```python
from build123d import *

# Parameters (mm, degrees)
F0_W     = 24
F0_H     = 12
F0_W_2   = 19.8
F0_H_2   = 3.2
F1_DEPTH = 0.9
F2_W     = 24
F2_H     = 12
F3_DEPTH = 2.7
F4_R     = 1.6
F5_DEPTH = 1.2
F6_R     = 0.2
F7_R     = 1.05
F8_DEPTH = 5


with BuildPart() as f1:
    # F0 (on Top) → F1 (new body)
    with BuildSketch(Plane.XY):
        Rectangle(F0_W, F0_H)
        with Locations((0, -2.35)):
            Rectangle(F0_W_2, F0_H_2, mode=Mode.SUBTRACT)
        with Locations((0, 2.35)):
            Rectangle(F0_W_2, F0_H_2, mode=Mode.SUBTRACT)
    extrude(amount=F1_DEPTH)

    # F2 (on face) → F3 (join)
    with BuildSketch(Plane(origin=(0, 0, 0), x_dir=(1, 0, 0), z_dir=(0, 0, -1))):
        Rectangle(F2_W, F2_H)
    extrude(amount=F3_DEPTH)

    # F4 (on face) → F5 (cut)
    with BuildSketch(Plane(origin=(0, 0, -2.7), x_dir=(1, 0, 0), z_dir=(0, 0, -1))):
        Circle(F4_R)
        with Locations((-9, 0)):
            Circle(F4_R)
        with Locations((9, 0)):
            Circle(F4_R)
    extrude(amount=-F5_DEPTH, mode=Mode.SUBTRACT)

    # F6
    f6_edges = [f1.edges().sort_by_distance(p)[0] for p in [
        (-12, -6, -0.9),
        (-12, 6, -0.9),
        (12, 6, -0.9),
        (12, -6, -0.9),
    ]]
    fillet(f6_edges, radius=F6_R)

    # F7 (on face) → F8 (cut)
    with BuildSketch(Plane.XZ.offset(6)):
        with Locations((-6.5, -1.15)):
            Circle(F7_R)
        with Locations((6.5, -1.15)):
            Circle(F7_R)
    extrude(amount=-F8_DEPTH, mode=Mode.SUBTRACT)


solid = f1.part
```
Can you work these out from the model? Positions are in its coordinate system, mm. A direction names the side the tool comes from. Round coordinates to 2 decimals unless told otherwise and drop trailing zeros. Loops run counter-clockwise (first coordinate to the right, second up) from the corner with the lowest first, then second, coordinate; pieces in that order, holes last. Notation, with made-up numbers: M 23.25,88 L 39.25,88 A30 cw 39.25,126 Z; hole C -19,-20.75 d11. An arc over 180 degrees is marked long. Write item = value, one per line. Start each with the question number.
(1) I need wall thicknesses on line 1 along Y through (x, z) = (0.75, 0.35); line 2 along X through (y, z) = (0, -2.3); line 3 along Y through (x, z) = (9, -1.9). Which ranges of each line are inside material? Lowest first, please.
(2) Which directions (+Z, -Z, +X, -X, +Y, -Y) give clear straight access to the entire face, cutting with the end or side of a thin tool? Please do faces 1 (the face through (-10.6, -0.07, -2.11)), 2 (the face through (6, -1, -1)), 3 (the face through (-0.1, -3.95, 0.4)).
(3) Suppose I cut it at A-A on y = 3.25. Write out the boundary of the cut face in (x, z), plus the area to 3 significant figures.
(4) Suppose I cut it at D-D on y = -5. Write out the boundary of the cut face in (x, z), plus the area to 3 significant figures.
(5) If we mould it in two halves opening along X, with no side actions, what happens to faces 4 (the face through (12, 0, -1)), 5 (the face through (-9.9, -2.4, 0.4)), 6 (the face through (-3, 0, -2.7))? For each: released by +X, released by -X, zero draft, split by the parting line, or undercut.
(6) Suppose I cut it at C-C on z = -1.8. Write out the boundary of the cut face in (x, y), plus the area to 3 significant figures.
(7) Suppose I cut it at B-B on x = -6.5. Write out the boundary of the cut face in (y, z).
Answer block:
q1.line_1 = -6 to -3.95, -0.75 to 0.75, 3.95 to 6
q1.line_2 = -12 to -10.6, -7.4 to -1.6, 1.6 to 7.4, 10.6 to 12
q1.line_3 = -6 to -1.6, 1.6 to 6
q2.face_1 = -Z
q2.face_2 = -Y
q2.face_3 = +Z
q3.outline = M -12,-2.7 L 12,-2.7 L 12,0.9 L 9.9,0.9 L 9.9,0 L -9.9,0 L -9.9,0.9 L -12,0.9 Z
q3.area = 68.6 mm²
q4.outline = M -12,-2.7 L 12,-2.7 L 12,0.9 L -12,0.9 Z; hole C -6.5,-1.15 d2.1; hole C 6.5,-1.15 d2.1
q4.area = 79.5 mm²
q5.face_4 = released by +X
q5.face_5 = undercut
q5.face_6 = zero draft
q6.outline = M -12,-5.8 A0.2 ccw -11.8,-6 L -7.32,-6 L -7.32,-1 L -5.68,-1 L -5.68,-6 L 5.68,-6 L 5.68,-1 L 7.32,-1 L 7.32,-6 L 11.8,-6 A0.2 ccw 12,-5.8 L 12,5.8 A0.2 ccw 11.8,6 L -11.8,6 A0.2 ccw -12,5.8 Z; hole C -9,0 d3.2; hole C 0,0 d3.2; hole C 9,0 d3.2
q6.area = 247 mm²
q7.outline = M -6,-2.7 L 6,-2.7 L 6,0.9 L 3.95,0.9 L 3.95,0 L 0.75,0 L 0.75,0.9 L -0.75,0.9 L -0.75,0 L -3.95,0 L -3.95,0.9 L -6,0.9 L -6,-0.1 L -1,-0.1 L -1,-2.2 L -6,-2.2 Z
